Geometry: final body of the model. Coordinates: model frame, mm. A direction names the side the tool comes from. Round coordinates to 2 decimals unless told otherwise and drop trailing zeros. Loops run counter-clockwise (first coordinate to the right, second up) from the corner with the lowest first, then second, coordinate; pieces in that order, holes last. Notation, with made-up numbers: M -38.5,41 L 4.5,41 A24 ccw 4.5,55 Z; hole C 86,38 d6. An arc over 180 degrees is marked long. Answer as a JSON object with one key per item and string values.
from build123d import *

# Parameters (mm, degrees)
CROQUIS2_W                = 92
CROQUIS2_H                = 40
SALIENTE_EXTRUIR2_DEPTH   = 4
CROQUIS3_W                = 3
CROQUIS3_H                = 40
SALIENTE_EXTRUIR3_DEPTH   = 95
SALIENTE_EXTRUIR3_2_DEPTH = 95
CROQUIS4_W                = 3
CROQUIS4_H                = 40
SALIENTE_EXTRUIR4_DEPTH   = 4
REDONDEO1_R               = 3
CROQUIS5_W                = 92
CROQUIS5_H                = 3
SALIENTE_EXTRUIR5_DEPTH   = 45
REDONDEO2_R               = 3
CROQUIS6_W                = 22
CROQUIS6_H                = 30
CORTAR_EXTRUIR1_DEPTH     = 26
CROQUIS7_R                = 2
CORTAR_EXTRUIR2_DEPTH     = 10


with BuildPart() as part:
    # Croquis2 → Saliente-Extruir2 (new body)
    with BuildSketch(Plane.XY):
        Rectangle(CROQUIS2_W, CROQUIS2_H)
    extrude(amount=SALIENTE_EXTRUIR2_DEPTH)



with BuildPart() as body_2:
    # Croquis3 → Saliente-Extruir3 (new body)
    with BuildSketch(Plane.XY.offset(4)):
        with Locations((-47.5, 0)):
            Rectangle(CROQUIS3_W, CROQUIS3_H)
    extrude(amount=SALIENTE_EXTRUIR3_DEPTH)


with BuildPart() as body_3:
    # Croquis3 → Saliente-Extruir3 2 (new body)
    with BuildSketch(Plane.XY.offset(4)):
        with Locations((47.5, 0)):
            Rectangle(CROQUIS3_W, CROQUIS3_H)
    extrude(amount=SALIENTE_EXTRUIR3_2_DEPTH)


with BuildPart() as part_1:
    add(part.part)

    add(body_2.part)  # Saliente-Extruir4 merges body 2

    add(body_3.part)  # Saliente-Extruir4 merges body 3
    # Croquis4 → Saliente-Extruir4 (add)
    with BuildSketch(Plane(origin=(0, 0, 4), x_dir=(-1, 0, 0), z_dir=(0, 0, -1))):
        with Locations((-47.5, 0)):
            Rectangle(CROQUIS4_W, CROQUIS4_H)
        with Locations((47.5, 0)):
            Rectangle(CROQUIS4_W, CROQUIS4_H)
    extrude(amount=SALIENTE_EXTRUIR4_DEPTH)

    # Redondeo1
    redondeo1_edges = [part_1.edges().sort_by_distance(p)[0] for p in [
        (49, 0, 0),
        (-49, 0, 0),
    ]]
    fillet(redondeo1_edges, radius=REDONDEO1_R)

    # Croquis5 → Saliente-Extruir5 (add)
    with BuildSketch(Plane.XY.offset(4)):
        with Locations((0, 18.5)):
            Rectangle(CROQUIS5_W, CROQUIS5_H)
    extrude(amount=SALIENTE_EXTRUIR5_DEPTH)

    # Redondeo2
    redondeo2_edges = [part_1.edges().sort_by_distance(p)[0] for p in [
        (-48.121320344, 20, 0.878679656),
        (0, 20, 0),
        (48.121320344, 20, 0.878679656),
        (-49, 20, 51),
        (49, 20, 51),
    ]]
    fillet(redondeo2_edges, radius=REDONDEO2_R)

    # Croquis6 → Cortar-Extruir1 (cut)
    with BuildSketch(Plane(origin=(0, 0, 0), x_dir=(-1, 0, 0), z_dir=(0, 0, -1))):
        with Locations((0, 5)):
            Rectangle(CROQUIS6_W, CROQUIS6_H)
    extrude(amount=-CORTAR_EXTRUIR1_DEPTH, mode=Mode.SUBTRACT)

    # Croquis7 → Cortar-Extruir2 (cut)
    with BuildSketch(Plane(origin=(0, 0, 0), x_dir=(-1, 0, 0), z_dir=(0, 0, -1))):
        with Locations((5, -15)):
            Circle(CROQUIS7_R)
        with Locations((-5, -15)):
            Circle(CROQUIS7_R)
        with Locations((13.733587387, -10.3)):
            Circle(CROQUIS7_R)
        with Locations((-13.733587387, -10.3)):
            Circle(CROQUIS7_R)
        with Locations((13.8, -0.300220534)):
            Circle(CROQUIS7_R)
        with Locations((-13.8, -0.300220534)):
            Circle(CROQUIS7_R)
    extrude(amount=-CORTAR_EXTRUIR2_DEPTH, mode=Mode.SUBTRACT)


solid = part_1.part
1) Reachability of faces 1 (the flat face through (0, 19, 26)), 2 (the flat face through (-1, -14, 4)), 3 (the cylindrical face through (5, -13, 2)), 4 (the flat face through (11, 10, 3)) from +Z, -Z, +X, -X, +Y, -Y: full face, straight path, thin tool, end or side. Return the list, or none.
Results:
{"face 1": "-Z, +Y, -Y", "face 2": "+Z, -Y", "face 3": "+Z, -Z", "face 4": "-Z, +Y"}
2) Section query A-A (y = 15). Return the cut outline in (x, z).
Results:
{"outline": "M -49,3 A3 ccw -46,0 L -11,0 L -11,4 L -46,4 L -46,99 L -49,99 Z; M 11,0 L 46,0 A3 ccw 49,3 L 49,99 L 46,99 L 46,4 L 11,4 Z"}
3) Pin query (flat end, axial travel): P1, Ø0.9, axis at x = -15, y = 19, coming from the +Z side; P2, Ø11, axis at x = 22.5, y = -9, coming from the +Z side; P3, Ø4.5, axis at x = 3.5, z = 1, coming from the +Y side. Return the tip coordinate at first contact, or that it passes through.
Results:
{"P1": "z = 49", "P2": "z = 4", "P3": "y = -10"}
4) Section query B-B (z = 57.5). Return the cut outline in (x, y), and give its area (3 significant figures).
Results:
{"outline": "M -49,-20 L -46,-20 L -46,20 A3 ccw -49,17 Z; M 46,-20 L 49,-20 L 49,17 A3 ccw 46,20 Z", "area": "236 mm2"}
5) Section query D-D (y = -15). Return the cut outline in (x, z), and give its area (3 significant figures).
Results:
{"outline": "M -49,3 A3 ccw -46,0 L -7,0 L -7,4 L -46,4 L -46,99 L -49,99 Z; M -3,0 L 3,0 L 3,4 L -3,4 Z; M 7,0 L 46,0 A3 ccw 49,3 L 49,99 L 46,99 L 46,4 L 7,4 Z", "area": "926 mm2"}
6) Section query C-C (x = 5). Return the cut outline in (y, z).
Results:
{"outline": "M -20,0 L -17,0 L -17,4 L -20,4 Z; M -13,0 L -10,0 L -10,4 L -13,4 Z; M 17,26 L 20,26 L 20,49 L 17,49 Z"}
7) Ray query, line 1 (Y direction, x = -13.8, z = 2.8); line 2 (X direction, y = -15, z = 83.5); line 3 (Y direction, x = 5, z = 3). Return the intervals inside material, ascending.
Results:
{"line 1": "-20 to -12.3, -8.3 to -2.3, 1.7 to 19.99", "line 2": "-49 to -46, 46 to 49", "line 3": "-20 to -17, -13 to -10"}
